Here's how the part is built. I have some questions about the finished solid (model axes, mm). A direction names the side the tool comes from. Round coordinates to 2 decimals unless told otherwise and drop trailing zeros. Order: outer loops, then holes, each group sorted by start corner. A loop starts at its lowest first (then second) coordinate and runs counter-clockwise, first axis right, second up. Notation, with made-up numbers: (-25, 44.5) - (30, 44.5) arc R13 cw to (30, 53.5) - close; hole circle Ø8 at (-37, 30.5). An arc over 180 degrees is marked (long way). One line per item, written item: value.
from build123d import *

# Parameters (mm, degrees)
SKETCH_1_W          = 82
SKETCH_1_H          = 82
SKETCH_1_R          = 1.75
EXTRUDE_1_DEPTH     = 2
CUT_EXTRUDE_START   = -2
SKETCH_2_R          = 1.75
SKETCH_2_R_2        = 0.8
SKETCH_2_R_3        = 1.2
CUT_EXTRUDE_1_DEPTH = 2
EXTRUDE_START       = -7
SKETCH_4_R          = 2
SKETCH_4_R_2        = 0.8
EXTRUDE_2_DEPTH     = 7
EXTRUDE_START_2     = -5
SKETCH_5_R          = 3
SKETCH_5_R_2        = 1.2
EXTRUDE_3_DEPTH     = 5
EXTRUDE_START_3     = -8
SKETCH_6_R          = 3
SKETCH_6_R_2        = 1.2
SKETCH_6_R_3        = 1.158828733
EXTRUDE_4_DEPTH     = 8
CUT_EXTRUDE_2_REACH = 82.589
SKETCH_7_W          = 82
SKETCH_7_H          = 82
SKETCH_7_W_2        = 81.6
SKETCH_7_H_2        = 81.6


with BuildPart() as part:
    # 草圖1 → 填料-伸長1 (new body)
    with BuildSketch(Plane(origin=(0, 0, 0), x_dir=(1, 0, 0), z_dir=(0, 1, 0))):
        with Locations((-4.734930226, -24.870201097)):
            Rectangle(SKETCH_1_W, SKETCH_1_H)
        with Locations(Location((-40.734930226, 11.129798903, 0), (0, 0, 270))):
            Circle(SKETCH_1_R, mode=Mode.SUBTRACT)
        with Locations(Location((-40.734930226, -60.870201097, 0), (0, 0, 270))):
            Circle(SKETCH_1_R, mode=Mode.SUBTRACT)
        with Locations(Location((31.265069774, 3.129798903, 0), (0, 0, 270))):
            Circle(SKETCH_1_R, mode=Mode.SUBTRACT)
        with Locations(Location((31.265069774, -60.870201097, 0), (0, 0, 270))):
            Circle(SKETCH_1_R, mode=Mode.SUBTRACT)
    extrude(amount=EXTRUDE_1_DEPTH)

    # 草圖2 → 除料-伸長1 (cut)
    with BuildSketch(Plane(origin=(0, 2, 0), x_dir=(1, 0, 0), z_dir=(0, 1, 0)).offset(CUT_EXTRUDE_START)):
        with Locations(Location((-40.734930226, 11.129798903, 0), (0, 0, 270))):
            Circle(SKETCH_2_R)
        with Locations(Location((-34.514930226, -14.570201097, 0), (0, 0, 270))):
            Circle(SKETCH_2_R_2)
        with Locations(Location((31.265069774, -14.570201097, 0), (0, 0, 270))):
            Circle(SKETCH_2_R_2)
        with Locations(Location((-33.734930226, -27.820201097, 0), (0, 0, 270))):
            Circle(SKETCH_2_R_3)
        with Locations(Location((-33.734930226, -61.870201097, 0), (0, 0, 270))):
            Circle(SKETCH_2_R_3)
        with Locations(Location((-9.684930226, -27.820201097, 0), (0, 0, 270))):
            Circle(SKETCH_2_R_3)
        with Locations(Location((-9.684930226, -61.870201097, 0), (0, 0, 270))):
            Circle(SKETCH_2_R_3)
        with Locations(Location((-0.734896325, -26.870201097, 0), (0, 0, 270))):
            Circle(SKETCH_2_R_3)
        with Locations(Location((24.265069774, -26.82902983, 0), (0, 0, 270))):
            Circle(SKETCH_2_R_3)
        with Locations(Location((-0.734896325, -61.870201097, 0), (0, 0, 270))):
            Circle(SKETCH_2_R_3)
        with Locations(Location((24.265069774, -61.82902983, 0), (0, 0, 270))):
            Circle(SKETCH_2_R_3)
        with Locations(Location((31.265069774, 11.129798903, 0), (0, 0, 270))):
            Circle(SKETCH_2_R_2)
        with Locations(Location((-34.514930226, 11.129798903, 0), (0, 0, 270))):
            Circle(SKETCH_2_R_2)
    extrude(amount=CUT_EXTRUDE_1_DEPTH, mode=Mode.SUBTRACT)

    # 草圖4 → 填料-伸長2 (add)
    # profile 1 of 4: a face of its own
    with BuildSketch(Plane(origin=(0, 2, 0), x_dir=(1, 0, 0), z_dir=(0, 1, 0)).offset(EXTRUDE_START)):
        with Locations(Location((-34.514930226, 11.129798903, 0), (0, 0, 270))):
            Circle(SKETCH_4_R)
        with Locations(Location((-34.514930226, 11.129798903, 0), (0, 0, 270))):
            Circle(SKETCH_4_R_2, mode=Mode.SUBTRACT)
    # profile 2 of 4: a face of its own
    with BuildSketch(Plane(origin=(0, 2, 0), x_dir=(1, 0, 0), z_dir=(0, 1, 0)).offset(EXTRUDE_START)):
        with Locations(Location((-34.514930226, -14.570201097, 0), (0, 0, 270))):
            Circle(SKETCH_4_R)
        with Locations(Location((-34.514930226, -14.570201097, 0), (0, 0, 270))):
            Circle(SKETCH_4_R_2, mode=Mode.SUBTRACT)
    # profile 3 of 4: a face of its own
    with BuildSketch(Plane(origin=(0, 2, 0), x_dir=(1, 0, 0), z_dir=(0, 1, 0)).offset(EXTRUDE_START)):
        with Locations(Location((31.265069774, 11.129798903, 0), (0, 0, 270))):
            Circle(SKETCH_4_R)
        with Locations(Location((31.265069774, 11.129798903, 0), (0, 0, 270))):
            Circle(SKETCH_4_R_2, mode=Mode.SUBTRACT)
    # profile 4 of 4: a face of its own
    with BuildSketch(Plane(origin=(0, 2, 0), x_dir=(1, 0, 0), z_dir=(0, 1, 0)).offset(EXTRUDE_START)):
        with Locations(Location((31.265069774, -14.570201097, 0), (0, 0, 270))):
            Circle(SKETCH_4_R)
        with Locations(Location((31.265069774, -14.570201097, 0), (0, 0, 270))):
            Circle(SKETCH_4_R_2, mode=Mode.SUBTRACT)
    extrude(amount=EXTRUDE_2_DEPTH)

    # 草圖5 → 填料-伸長3 (add)
    # profile 1 of 4: a face of its own
    with BuildSketch(Plane(origin=(0, 2, 0), x_dir=(1, 0, 0), z_dir=(0, 1, 0)).offset(EXTRUDE_START_2)):
        with Locations(Location((-33.734930226, -27.820201097, 0), (0, 0, 270))):
            Circle(SKETCH_5_R)
        with Locations(Location((-33.734930226, -27.820201097, 0), (0, 0, 270))):
            Circle(SKETCH_5_R_2, mode=Mode.SUBTRACT)
    # profile 2 of 4: a face of its own
    with BuildSketch(Plane(origin=(0, 2, 0), x_dir=(1, 0, 0), z_dir=(0, 1, 0)).offset(EXTRUDE_START_2)):
        with Locations(Location((-9.684930226, -27.820201097, 0), (0, 0, 270))):
            Circle(SKETCH_5_R)
        with Locations(Location((-9.684930226, -27.820201097, 0), (0, 0, 270))):
            Circle(SKETCH_5_R_2, mode=Mode.SUBTRACT)
    # profile 3 of 4: a face of its own
    with BuildSketch(Plane(origin=(0, 2, 0), x_dir=(1, 0, 0), z_dir=(0, 1, 0)).offset(EXTRUDE_START_2)):
        with Locations(Location((-33.734930226, -61.870201097, 0), (0, 0, 270))):
            Circle(SKETCH_5_R)
        with Locations(Location((-33.734930226, -61.870201097, 0), (0, 0, 270))):
            Circle(SKETCH_5_R_2, mode=Mode.SUBTRACT)
    # profile 4 of 4: a face of its own
    with BuildSketch(Plane(origin=(0, 2, 0), x_dir=(1, 0, 0), z_dir=(0, 1, 0)).offset(EXTRUDE_START_2)):
        with Locations(Location((-9.684930226, -61.870201097, 0), (0, 0, 270))):
            Circle(SKETCH_5_R)
        with Locations(Location((-9.684930226, -61.870201097, 0), (0, 0, 270))):
            Circle(SKETCH_5_R_2, mode=Mode.SUBTRACT)
    extrude(amount=EXTRUDE_3_DEPTH)

    # 草圖6 → 填料-伸長4 (add)
    # profile 1 of 4: a face of its own
    with BuildSketch(Plane(origin=(0, 2, 0), x_dir=(1, 0, 0), z_dir=(0, 1, 0)).offset(EXTRUDE_START_3)):
        with Locations(Location((-0.734896325, -26.870201097, 0), (0, 0, 270))):
            Circle(SKETCH_6_R)
        with Locations(Location((-0.734896325, -26.870201097, 0), (0, 0, 270))):
            Circle(SKETCH_6_R_2, mode=Mode.SUBTRACT)
    # profile 2 of 4: a face of its own
    with BuildSketch(Plane(origin=(0, 2, 0), x_dir=(1, 0, 0), z_dir=(0, 1, 0)).offset(EXTRUDE_START_3)):
        with Locations(Location((24.265069774, -26.82902983, 0), (0, 0, 270))):
            Circle(SKETCH_6_R)
        with Locations(Location((24.265069774, -26.82902983, 0), (0, 0, 270))):
            Circle(SKETCH_6_R_2, mode=Mode.SUBTRACT)
    # profile 3 of 4: a face of its own
    with BuildSketch(Plane(origin=(0, 2, 0), x_dir=(1, 0, 0), z_dir=(0, 1, 0)).offset(EXTRUDE_START_3)):
        with Locations(Location((-0.734896325, -61.870201097, 0), (0, 0, 270))):
            Circle(SKETCH_6_R)
        with Locations(Location((-0.734896325, -61.870201097, 0), (0, 0, 270))):
            Circle(SKETCH_6_R_2, mode=Mode.SUBTRACT)
    # profile 4 of 4: a face of its own
    with BuildSketch(Plane(origin=(0, 2, 0), x_dir=(1, 0, 0), z_dir=(0, 1, 0)).offset(EXTRUDE_START_3)):
        with Locations(Location((24.265069774, -61.870201097, 0), (0, 0, 270))):
            Circle(SKETCH_6_R)
        with Locations(Location((24.265069774, -61.870201097, 0), (0, 0, 270))):
            Circle(SKETCH_6_R_3, mode=Mode.SUBTRACT)
    extrude(amount=EXTRUDE_4_DEPTH)

    # 草圖7 → 除料-伸長2 (cut, up to next)
    with BuildSketch(Plane(origin=(0, 2, 0), x_dir=(1, 0, 0), z_dir=(0, 1, 0)), mode=Mode.PRIVATE) as cut_extrude_2_sk1:
        with Locations((-4.734930226, -24.870201097)):
            Rectangle(SKETCH_7_W, SKETCH_7_H)
        with Locations((-4.734930226, -24.870201097)):
            Rectangle(SKETCH_7_W_2, SKETCH_7_H_2, mode=Mode.SUBTRACT)
    cut_extrude_2_tool1 = extrude(cut_extrude_2_sk1.sketch, amount=-CUT_EXTRUDE_2_REACH, mode=Mode.PRIVATE) & part.part
    add(cut_extrude_2_tool1.solids().sort_by_distance((-4.73493, 2, -16.013833))[0], mode=Mode.SUBTRACT)


solid = part.part
Q1. If we section it at A-A, the plane y = -4: Give the number of separate pieces and of enclosed holes in the cut face, then the cut area to 3 significant figures.
Results list:
separate pieces: 8
enclosed holes: 8
area: 138 mm²
Q2. Which directions (+Z, -Z, +X, -X, +Y, -Y) give clear straight access to the entire face, cutting with the end or side of a thin tool? Please do faces 4 (the cylindrical face through (24, -2, 28)), 5 (the cylindrical face through (29.49, -2.54, -10.21)).
Results list:
face 4: +Y, -Y
face 5: -Y
Q3. Will these pins go through, and if not, where does the flat tip stop? pin 1 (4 mm diameter, centred on x = 31.27, z = -3.13, fed in from -Y); pin 2 (1.8 mm diameter, centred on x = 31.27, z = -11.13, fed in from -Y); pin 3 (4 mm diameter, centred on x = -33.73, z = 27.82, fed in from -Y); pin 4 (2 mm diameter, centred on x = -9.68, z = 27.82, fed in from -Y).
Results list:
pin 1: y = 0
pin 2: y = -5
pin 3: y = -3
pin 4: through
Q4. We'd pull the mould along X, two halves only. Please class faces 1 (the flat face through (-45.535, 1, 25)), 2 (the flat face through (-34, -5, -10)), 3 (the cylindrical face through (-33.374, -0.535, 28.965)): released by +X, released by -X, zero draft, split by the parting line, or undercut.
Results list:
face 1: released by -X
face 2: zero draft
face 3: undercut
Q5. If we section it at B-B, the plane x = 10: Please give me the cut outline in (y, z).
Results list:
outline: (0, -15.93) - (2, -15.93) - (2, 65.67) - (0, 65.67) - close
Q6. If we section it at C-C, the plane z = 8.5: Please give me the cut outline in (x, y), then the cut area to 3 significant figures.
Results list:
outline: (-45.53, 0) - (36.07, 0) - (36.07, 2) - (-45.53, 2) - close
area: 163 mm²
Q7. If I drill on line 1 along X through (y, z) = (-2.25, 60.5); line 2 along Z through (x, y) = (31, -1); line 3 along X through (y, z) = (-1.25, 60), over which ranges is the centre line in solid material (lowest first)?
Results list:
line 1: -36.4 to -31.07, -12.35 to -7.02, -3.4 to 1.93, 21.6 to 26.93
line 2: -13.11 to -11.88, -10.37 to -9.15, 12.59 to 13.82, 15.33 to 16.55
line 3: -36.08 to -31.39, -12.03 to -7.34, -3.08 to 1.61, 21.92 to 26.61
